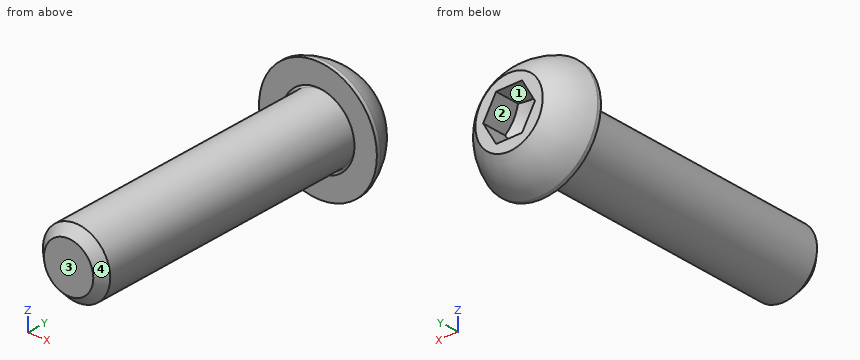
```python
from build123d import *

# Parameters (mm, degrees)
Y_KSEKLIK_EKSTR_ZYON1_START = -2.378633
IZIM2_R                     = 3
Y_KSEKLIK_EKSTR_ZYON1_DEPTH = 2.378633


with BuildPart() as part:
    # Çizim1 → Döndür1 (revolve)
    with BuildSketch(Plane.XY):
        with BuildLine():
            Line((2.309401077, 0), (3, 0))
            ThreePointArc((3, 0), (4.355337259, -1.310502077), (5.25, -2.97))
            Line((5.25, -2.97), (5.25, -3.3))
            Line((5.25, -3.3), (3.25, -3.3))
            ThreePointArc((3.25, -3.3), (3.426776695, -2.873223305), (3, -3.05))
            Line((3, -3.05), (3, -27.5))
            Line((3, -27.5), (2.2, -28.3))
            Line((2.2, -28.3), (0, -28.3))
            Line((0, -28.3), (0, -3.533333333))
            Line((0, -3.533333333), (2.309401077, -2.2))
            Line((2.309401077, -2.2), (2.309401077, 0))
        make_face()
    revolve(axis=Axis((0, -3.533333333, 0), (0, -1, 0)))

    # Çizim2 → Yükseklik-Ekstrüzyon1 (add)
    with BuildSketch(Plane(origin=(0, 0, 0), x_dir=(1, 0, 0), z_dir=(0, 1, 0)).offset(Y_KSEKLIK_EKSTR_ZYON1_START)):
        Circle(IZIM2_R)
        Polygon((2.309401077, 0), (1.154700538, 2), (-1.154700538, 2), (-2.309401077, 0), (-1.154700538, -2), (1.154700538, -2), align=None, mode=Mode.SUBTRACT)
    extrude(amount=Y_KSEKLIK_EKSTR_ZYON1_DEPTH)


solid = part.part
```
Model file for the job. Use its own axes, mm. Face numbers are marked on the shaded views. Give positions to 0.01 mm unless a question says otherwise; leave off trailing zeros. One line per question, with ' | ' between items. Start each with the question number.
(1) Two-plate mould, pull along X, no slides. Class the marked faces 1, 2, 3 and 4: +X half, -X half, draft (parallel to the pull), parting line (faces both ways), or undercut.
(2) Wall check: line 1 along Y through (x, z) = (0.75, 4.75); line 2 along Z through (x, y) = (-0.25, -4.25); line 3 along X through (y, z) = (-12.75, 1.5). Give the ranges that are in metal, low to high. Write a range as from..to.
(3) Pin check, flat tips, straight feed: P1, Ø1.2, axis at x = -0.5, y = -1.5, coming from the +Z side; P2, Ø4, axis at y = -25, z = 0.5, coming from the +X side; P3, Ø4, axis at x = 4, y = -22, coming from the -Z side. Stop position of each tip, or through.
Results below:
1) face 1: undercut | face 2: undercut | face 3: draft | face 4: parting line
2) line 1: -3.3..-2 | line 2: -2.99..2.99 | line 3: -2.6..2.6
3) P1: z = 4.84 | P2: x = 3 | P3: z = -2.24
